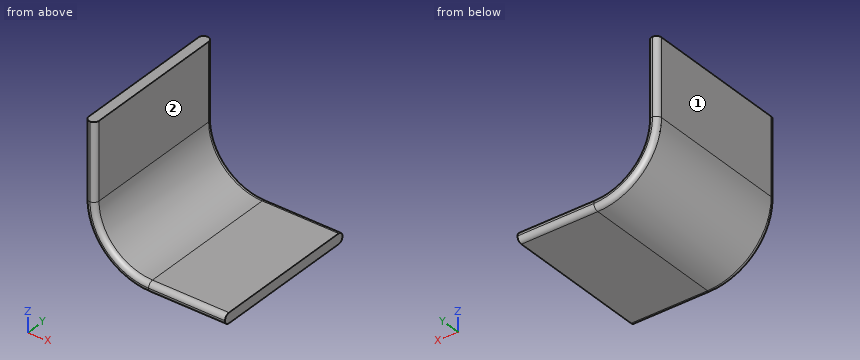
from build123d import *

# Parameters (mm, degrees)
BOSS_EXTRUDE1_DEPTH = 60
FILLET1_R           = 2


with BuildPart() as part:
    # Sketch1 → Boss-Extrude1 (new body)
    with BuildSketch(Plane(origin=(0, 0, 0), x_dir=(1, 0, 0), z_dir=(0, 1, 0))):
        with BuildLine():
            Line((-25, 0), (-25, -15))
            Line((-25, -15), (-25, -30))
            Line((-25, -30), (-21, -30))
            Line((-21, -30), (-21, -15))
            Line((-21, -15), (-21, 0))
            ThreePointArc((-21, 0), (-14.849242405, 14.849242405), (0, 21))
            Line((0, 21), (15, 21))
            Line((15, 21), (30, 21))
            Line((30, 21), (30, 25))
            Line((30, 25), (15, 25))
            Line((15, 25), (0, 25))
            ThreePointArc((0, 25), (-17.67766953, 17.67766953), (-25, 0))
        make_face()
    extrude(amount=BOSS_EXTRUDE1_DEPTH)

    # Fillet1
    fillet1_edges = [part.edges().sort_by_distance(p)[0] for p in [
        (15, 0, -25),
        (-25, 0, 15),
        (-21, 0, 15),
        (15, 0, -21),
        (15, 60, -25),
        (-25, 60, 15),
        (-21, 60, 15),
        (15, 60, -21),
        (-17.67766953, 0, -17.67766953),
        (-14.849242405, 0, -14.849242405),
        (-17.67766953, 60, -17.67766953),
        (-14.849242405, 60, -14.849242405),
    ]]
    fillet(fillet1_edges, radius=FILLET1_R - 0.0001)  # a hair under: the kernel refuses the full size


solid = part.part
CAD build for the part. Positions are in the model's coordinates, mm. Face numbers are marked on the shaded views. A direction names the side the tool comes from. Round coordinates to 2 decimals unless told otherwise and drop trailing zeros. Write each loop counter-clockwise with the first axis right and the second up, starting at its lowest first coordinate (ties: lowest second). Pieces come first, ordered by that corner, then holes. Notation, with made-up numbers: M 8.25,-38 L 22.25,-38 A35 ccw 22.25,-6 Z; hole C -7.5,8 d10. An arc over 180 degrees is marked long. Use a Markdown table: item, result. Add a question column.
1. Drill centre lines: probe 1 along Z at (x, y) = (27.5, 35.5); probe 2 along Z at (x, y) = (-7, 40.5). Where is each one in solid material? Low to high.
2. Slice it at A-A on y = 11. Give the cut face in (x, z), then the cut area to 3 significant figures.
3. 3-axis set-ups, long thin cutter, end or side, ignore diameter. For the marked faces 1 and 2: which of +Z, -Z, +X, -X, +Y, -Y reach the whole face in a straight line?
4. Flat gauge pins, fed straight in: P1, Ø8, axis at x = 8, y = 12, coming from the +Z side; P2, Ø9, axis at y = 33, z = 17, coming from the +X side; P3, Ø5, axis at x = -8, y = 47, coming from the -Z side. Where does each tip first touch, or does it go through?
Reply:
| question | item | result |
|---|---|---|
| 1 | probe 1 | z = -25 to -21 |
| 1 | probe 2 | z = -24 to -19.8 |
| 2 | outline | M -25,0 A25 ccw 0,-25 L 30,-25 L 30,-21 L 0,-21 A21 cw -21,0 L -21,30 L -25,30 Z |
| 2 | area | 385 mm^2 |
| 3 | face 1 | +Z, -Z, -X, +Y, -Y |
| 3 | face 2 | +Z, +X, +Y, -Y |
| 4 | P1 | stops at z = -21 |
| 4 | P2 | stops at x = -21 |
| 4 | P3 | stops at z = -24.39 |
